from build123d import *

# Parameters (mm, degrees)
SKETCH_1_W           = 19
SKETCH_1_H           = 10
SKETCH_1_W_2         = 70
SKETCH_1_H_2         = 35
EXTRUDE_1_DEPTH      = 42
SKETCH_2_W           = 6.5
SKETCH_2_H           = 18
CUT_EXTRUDE_1_DEPTH  = 87.140872993
SKETCH_3_W           = 20
SKETCH_3_H           = 21
SKETCH_3_W_2         = 12
SKETCH_3_H_2         = 14
CUT_EXTRUDE_2_DEPTH  = 4
EXTRUDE_2_DEPTH      = 4
EXTRUDE_2_DEPTH_BACK = 4


with BuildPart() as part:
    # Эскиз1 → Бобышка-Вытянуть1 (new body)
    with BuildSketch(Plane.XY):
        with Locations((0, -22.5)):
            Rectangle(SKETCH_1_W, SKETCH_1_H)
        Rectangle(SKETCH_1_W_2, SKETCH_1_H_2)
    extrude(amount=EXTRUDE_1_DEPTH)

    # Эскиз2 → Вырез-Вытянуть1 (cut, through all)
    with BuildSketch(Plane(origin=(35, 0, 0), x_dir=(0, 0, -1), z_dir=(1, 0, 0))):
        with Locations((-3.25, 0)):
            Rectangle(SKETCH_2_W, SKETCH_2_H)
    extrude(amount=-CUT_EXTRUDE_1_DEPTH, mode=Mode.SUBTRACT)

    # Эскиз3 → Вырез-Вытянуть2 (cut)
    with BuildSketch(Plane.XY.offset(42)):
        with Locations((25, 0)):
            Rectangle(SKETCH_3_W, SKETCH_3_H)
        with Locations((-29, 0)):
            Rectangle(SKETCH_3_W_2, SKETCH_3_H_2)
    extrude(amount=-CUT_EXTRUDE_2_DEPTH, mode=Mode.SUBTRACT)

    # Эскиз4 → Бобышка-Вытянуть2 (add, two sides: drawn at the far end of the back side and taken through both)
    with BuildSketch(Plane(origin=(0, 0, 0), x_dir=(0, 0, -1), z_dir=(1, 0, 0)).offset(-EXTRUDE_2_DEPTH_BACK)):
        Polygon((-48, -13.5), (-42, -13.5), (-42, 3.5), (-45, 3.5), (-48, -7.5), align=None)
    extrude(amount=EXTRUDE_2_DEPTH + EXTRUDE_2_DEPTH_BACK)


solid = part.part
Verification items for the finished model (mm, model axes). A direction names the side the tool comes from. Round coordinates to 2 decimals unless told otherwise and drop trailing zeros. Loops run counter-clockwise (first coordinate to the right, second up) from the corner with the lowest first, then second, coordinate; pieces in that order, holes last. Notation, with made-up numbers: (-15, -29) - (-10, -29) arc R22 ccw to (-10, 5) - close; hole circle Ø8 at (-15.5, -40). An arc over 180 degrees is marked (long way). Write item = value, one per line.
Q1. Sectioned sample at C-C on y = 1.5. Record the boundary of the cut face in (x, z).
Here are the results:
outline = (-35, 6.5) - (35, 6.5) - (35, 38) - (15, 38) - (15, 42) - (4, 42) - (4, 45.55) - (-4, 45.55) - (-4, 42) - (-23, 42) - (-23, 38) - (-35, 38) - close
Q2. Depth check by flat-ended pin: pin 1 (12 mm diameter, centred on x = 19.5, y = -1, fed in from +Z); pin 2 (5 mm diameter, centred on x = -4, y = 1.5, fed in from -Z); pin 3 (22.5 mm diameter, centred on x = -7.5, y = 3, fed in from +Z); pin 4 (3 mm diameter, centred on y = -24.5, z = 28.5, fed in from +X). Enter the tip coordinate at first touch or a pass-through.
Here are the results:
pin_1 = 42
pin_2 = 6.5
pin_3 = 48
pin_4 = 9.5
Q3. Tool access check on faces 5 (the flat face through (0, 0, 6.5)), 6 (the flat face through (0, 3.5, 43)), 7 (the flat face through (-29, -7, 40)), 8 (the flat face through (25, 10.5, 40)), 9 (the flat face through (4, -5, 44)). Record the directions out of +Z, -Z, +X, -X, +Y, -Y that give a thin tool (end or side, any length) a straight path to the whole face; none if there is none.
Here are the results:
face_5 = -Z, +X, -X
face_6 = +Z, +X, -X, +Y
face_7 = +Z, -X
face_8 = +Z, +X
face_9 = +Z, +X, +Y, -Y
Q4. Sectioned sample at D-D on z = 24. Record the boundary of the cut face in (x, y).
Here are the results:
outline = (-35, -17.5) - (-9.5, -17.5) - (-9.5, -27.5) - (9.5, -27.5) - (9.5, -17.5) - (35, -17.5) - (35, 17.5) - (-35, 17.5) - close
Q5. Sectioned sample at A-A on z = 41. Record the boundary of the cut face in (x, y), plus the area to 3 significant figures.
Here are the results:
outline = (-35, -17.5) - (-9.5, -17.5) - (-9.5, -27.5) - (9.5, -27.5) - (9.5, -17.5) - (35, -17.5) - (35, -10.5) - (15, -10.5) - (15, 10.5) - (35, 10.5) - (35, 17.5) - (-35, 17.5) - (-35, 7) - (-23, 7) - (-23, -7) - (-35, -7) - close
area = 2,050 mm^2
Q6. Material ranges on L1, parallel to Y at x = 10.5, z = 4; L2, parallel to Y at x = -11.5, z = 9; L3, parallel to Y at x = -29, z = 39, recorded low to high.
Here are the results:
L1 = -17.5 to -9, 9 to 17.5
L2 = -17.5 to 17.5
L3 = -17.5 to -7, 7 to 17.5
Q7. Sectioned sample at B-B on x = 10.5. Record the boundary of the cut face in (y, z), plus the area to 3 significant figures.
Here are the results:
outline = (-17.5, 0) - (-9, 0) - (-9, 6.5) - (9, 6.5) - (9, 0) - (17.5, 0) - (17.5, 42) - (-17.5, 42) - close
area = 1,350 mm^2
Q8. Mould release check, pull along Y, two halves, no side actions. Record for faces 1 (the flat face through (-23, 0, 40)), 2 (the flat face through (0, -13.5, 45)), 3 (the flat face through (-35, 0, 21)), 4 (the flat face through (25, 0, 38)): +Y half, -Y half, draft (parallel to the pull), parting line (faces both ways), or undercut.
Here are the results:
face_1 = undercut
face_2 = -Y half
face_3 = draft
face_4 = undercut
